The model under review builds one solid part; all positions refer to its coordinate system, in mm. A direction names the side the tool comes from. Round coordinates to 2 decimals unless told otherwise and drop trailing zeros. Order: outer loops, then holes, each group sorted by start corner. A loop starts at its lowest first (then second) coordinate and runs counter-clockwise, first axis right, second up. Notation, with made-up numbers: M -29,8.5 L 7,8.5 A18 ccw 7,22.5 Z; hole C -37,44 d4. An arc over 180 degrees is marked long. Use a Markdown table: item, result. Add a question column.
1. To check wall thickness, follow probe 1 along Z at (x, y) = (0, 7.5); probe 2 along Y at (x, z) = (-5.5, 59); probe 3 along Y at (x, z) = (47, -30). State the ranges of each line that lie inside material, in increasing order.
2. Consider section D-D on y = 108.5. State the section outline as (x, z) points.
3. Consider section A-A on z = 0. State the section outline as (x, y) points, then the cut area to 3 significant figures.
4. Insertion check: P1, Ø2, axis at x = -49, z = -14, coming from the +Y side; P2, Ø1, axis at x = -29.5, z = 32.5, coming from the +Y side; P3, Ø4, axis at y = 47, z = -31, coming from the -X side. Each pin has a flat end and moves straight along its axis. Give the tip position at first contact, or say it passes through.
5. Consider section B-B on z = 57. Count the separate pieces of the cut face and the enclosed holes in it, then the cut area to 3 significant figures.
6. For faces 1 (the cylindrical face through (-38, 5.58, -35.87)), 2 (the cylindrical face through (-3.255, 96.787, 53.004)), 3 (the cylindrical face through (-0.651, 5.577, 52.043)), list the 3-axis set-ups (+Z, -Z, +X, -X, +Y, -Y) from which the entire face can be reached by the end or side of a thin tool; tool diameter is ignored.
7. The part is to be moulded in two halves that separate along X. For faces 4 (the cylindrical face through (53.57, 5.58, -41.07)), 5 (the flat face through (15, 12, 45)), 6 (the cylindrical face through (-37.6, 5.6, 36.1)), say which applies: +X half, -X half, draft (parallel to the pull), parting line (faces both ways), or undercut.
Autodesk Inventor part; units mm, degrees
ref_plane "Pracovní rovina1" through (0, 0, 67.5) normal (0, 0, 1) x (1, 0, 0)
ref_plane "YZ Plane" through (0, 0, 0) normal (1, 0, 0) x (0, 1, 0)
ref_plane "XZ Plane" through (0, 0, 0) normal (0, 1, 0) x (-1, 0, 0)
sketch "Náčrt1" plane through (0, 0, 0) normal (0, 0, 1) x (1, 0, 0)
  line L0 (-40.537, 0) -> (-67.5, 0)
  line L1 (-67.5, 0) -> (-67.5, 12)
  line L2 (-67.5, 12) -> (-42.4986, 12)
  line L3 (-42.4986, 12) -> (-32, 132)
  line L4 (-32, 132) -> (-28.9885, 132)
  line L5 (-28.9885, 132) -> (-40.537, 0)
  line L6 (-81, 0) -> (13.5, 0)
  line L7 (0, -26.4) -> (0, 158.4)
  point P0 (0, 0)
  dimension "d0" = 12
  dimension "d1" = 132
  dimension "d2" = 32
  dimension "d4" = 3
  dimension "d5" = 67.5
  dimension "d6" = 5
  dimension "d7" = 0
revolve "Rotace1" add sketch "Náčrt1" angle 360 about axis through (0, -10, 0) along (0, 1, 0)
sketch "Náčrt2" plane through (0, 12, 0) normal (0, 1, 0) x (1, 0, 0)
  circle A0 centre (0, 0) radius 57 construction
  line L0 (0, 94.5) -> (0, -94.5) construction
  line L1 (-94.5, 0) -> (94.5, 0) construction
  circle A1 centre (0, 57) radius 5
  circle A2 centre (-40.3051, 40.3051) radius 5
  circle A3 centre (-57, 0) radius 5
  circle A4 centre (-40.3051, -40.3051) radius 5
  circle A5 centre (0, -57) radius 5
  circle A6 centre (40.3051, -40.3051) radius 5
  circle A7 centre (57, 0) radius 5
  circle A8 centre (40.3051, 40.3051) radius 5
  dimension "d9" = 114
  dimension "d11" = 10
  dimension "d14" = 360
extrude "Vysunutí1" cut sketch "Náčrt2" against normal through all
chamfer "Zkosení1" distance 1 angle 45 9 edges at (-62, 12, 0) (-45.3051, 12, 40.3051) (-5, 12, 57) (35.3051, 12, 40.3051) (52, 12, 0) (35.3051, 12, -40.3051) (-5, 12, -57) (-45.3051, 12, -40.3051) (67.5, 12, 0)
ref_plane "Pracovní rovina1" through (0, 0, 67.5) normal (0, 0, 1) x (1, 0, 0)
sketch "Náčrt3" plane through (0, 0, 67.5) normal (0, 0, 1) x (1, 0, 0)
  line L0 (0, -26.4) -> (0, 158.4) construction
  line L1 (-94.5, 0) -> (94.5, 0) construction
  circle A0 centre (0, 72) radius 25
  point P0 (0, 0)
  dimension "d22" = 50
  dimension "d23" = 72
extrude "Vysunutí2" add sketch "Náčrt3" against normal up to next
sketch "Náčrt4" plane through (0, 72, 67.5) normal (0, 0, 1) x (1, 0, 0)
  circle A0 centre (0, 0) radius 25
  circle A1 centre (0, 0) radius 23.5
  point P0 (0, -72)
  dimension "d27" = 47
extrude "Vysunutí3" cut sketch "Náčrt4" against normal up to next contours A1
fillet "Zaoblení1" radius 5 2 edges at (-24.9752, 70.8872, 27.7671) (42.4986, 12, 0)
properties part number "Součást12"
Answer block:
| question | item | result |
|---|---|---|
| 1 | probe 1 | -67.5 to -62, -52 to -39.88, 39.88 to 52, 62 to 67.5 |
| 1 | probe 2 | 0 to 11.85, 47.61 to 49.15, 94.85 to 96.39 |
| 1 | probe 3 | 0 to 12 |
| 2 | outline | C 0,0 d68.11; hole C 0,0 d62.09 |
| 3 | outline | M -67.5,0 L -62,0 L -62,11 L -63,12 L -66.5,12 L -67.5,11 Z; M -52,0 L -40.54,0 L -28.99,132 L -32,132 L -42.1,16.56 A5 cw -47.08,12 L -51,12 L -52,11 Z; M 28.99,132 L 40.54,0 L 52,0 L 52,11 L 51,12 L 47.08,12 A5 cw 42.1,16.56 L 32,132 Z; M 62,0 L 67.5,0 L 67.5,11 L 66.5,12 L 63,12 L 62,11 Z |
| 3 | area | 1,150 mm^2 |
| 4 | P1 | y = 12 |
| 4 | P2 | y = 13.62 |
| 4 | P3 | x = -26.74 |
| 5 | separate pieces | 3 |
| 5 | enclosed holes | 1 |
| 5 | area | 973 mm^2 |
| 6 | face 1 | +Y, -Y |
| 6 | face 2 | +Z |
| 6 | face 3 | -Y |
| 7 | face 4 | parting line |
| 7 | face 5 | draft |
| 7 | face 6 | undercut |
